Source: CAD feature listing. Evaluate the final solid. Frame: model axes, mm. Face numbers are marked on the shaded views. A direction names the side the tool comes from. Give positions to 0.01 mm unless a question says otherwise; leave off trailing zeros. Order: outer loops, then holes, each group sorted by start corner. A loop starts at its lowest first (then second) coordinate and runs counter-clockwise, first axis right, second up. Notation, with made-up numbers: M 2,21 L 15,21 A16 cw 15,40 Z; hole C 26.5,55.25 d4. An arc over 180 degrees is marked long. Answer as a JSON object with one key per item and string values. Group by question number.
1. Section query C-C (x = -20). Output: boundary loops of the cut face in (y, z).
2. Section query B-B (y = -0.25). Output: boundary loops of the cut face in (x, z).
3. Section query A-A (z = 2.8). Output: boundary loops of the cut face in (x, y), plus the area to 3 significant figures.
4. Pin query (flat end, axial travel): P1, Ø1.5, axis at y = -12, z = 3, coming from the +X side; P2, Ø1, axis at x = 9.5, z = 2, coming from the -Y side; P3, Ø1.3, axis at x = -15, z = 1, coming from the +Y side. Return the tip coordinate at first contact, or that it passes through.
5. Section query D-D (y = -22.5). Output: boundary loops of the cut face in (x, z), plus the area to 3 significant figures.
6. Material intervals for L1, parallel to X at y = -6, z = 3.2; L2, parallel to X at y = -5.75, z = 0.3; L3, parallel to Y at x = -22, z = 2.9, sorted ascending. Write a range as [from, to].
7. Set-up query: the marked faces 1, 2 and 3. Return all of +Z, -Z, +X, -X, +Y, -Y with unobstructed straight access to the full face (end or side cutting, diameter ignored); none if empty.
from build123d import *

# Parameters (mm, degrees)
SKETCH1_R           = 25
SKETCH1_R_2         = 8
BASE_EXTRUDE_DEPTH  = 4.2
CUT_EXTRUDE1_DEPTH  = 5.2
BOSS_EXTRUDE1_DEPTH = 4.2


with BuildPart() as part:
    # Sketch1 → Base-Extrude (new body)
    with BuildSketch(Plane.XY):
        Circle(SKETCH1_R)
        Circle(SKETCH1_R_2, mode=Mode.SUBTRACT)
    extrude(amount=BASE_EXTRUDE_DEPTH)

    # Sketch2 → Cut-Extrude1 (cut, through all)
    with BuildSketch(Plane.XY.offset(4.2)):
        Polygon((-31.283198073, -2.2), (32.499555714, -2.2), (32.499555714, 32.618237466), (-31.739332188, 32.618237466), align=None)
    extrude(amount=-CUT_EXTRUDE1_DEPTH, mode=Mode.SUBTRACT)

    # Sketch3 → Boss-Extrude1 (add)
    with BuildSketch(Plane.XY.offset(4.2)):
        with BuildLine():
            Line((7.691553809, -2.2), (11.86423196, -2.2))
            ThreePointArc((11.86423196, -2.2), (9.256550998, -1.233150178), (7.909487973, 1.2))
            ThreePointArc((7.909487973, 1.2), (7.983616109, -0.511736089), (7.691553809, -2.2))
        make_face()
        with BuildLine():
            Line((-11.86423196, -2.2), (-7.691553809, -2.2))
            ThreePointArc((-7.691553809, -2.2), (-7.983616109, -0.511736089), (-7.909487973, 1.2))
            ThreePointArc((-7.909487973, 1.2), (-9.256550998, -1.233150178), (-11.86423196, -2.2))
        make_face()
    extrude(amount=-BOSS_EXTRUDE1_DEPTH)


solid = part.part
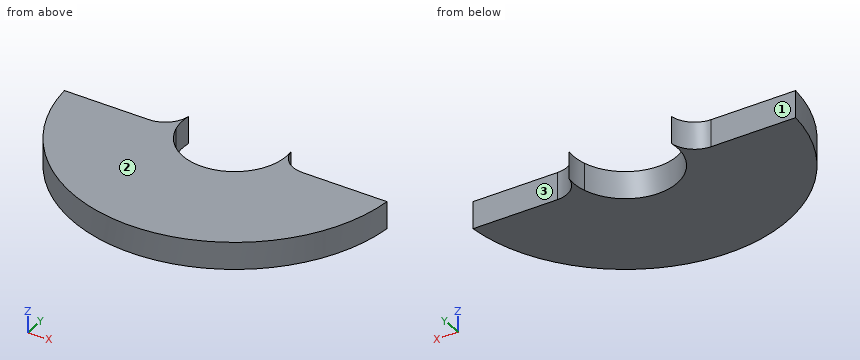
Answer sheet:
{
 "1": {"outline": "M -15,0 L -2.2,0 L -2.2,4.2 L -15,4.2 Z"},
 "2": {"outline": "M -8.43,0 L -8,0 L -8,4.2 L -8.43,4.2 Z; M 8,0 L 8.43,0 L 8.43,4.2 L 8,4.2 Z"},
 "3": {"outline": "M -24.9,-2.2 A25 ccw 24.9,-2.2 L 11.86,-2.2 A4 cw 7.91,1.2 A8 cw long -7.91,1.2 A4 cw -11.86,-2.2 Z", "area": "813 mm^2"},
 "4": {"P1": "x = 22.33", "P2": "y = -23.32", "P3": "y = -2.2"},
 "5": {"outline": "M -10.9,0 L 10.9,0 L 10.9,4.2 L -10.9,4.2 Z", "area": "91.5 mm^2"},
 "6": {"L1": "[-24.27, -5.29], [5.29, 24.27]", "L2": "[-24.33, -5.56], [5.56, 24.33]", "L3": "[-11.87, -2.2]"},
 "7": {"face 1": "+Z, -Z, -X, +Y", "face 2": "+Z, +X, -X, +Y, -Y", "face 3": "+Z, -Z, +X, +Y"}
}
